```python
from build123d import *
from build123d.topology import SkipClean

# Parameters (mm, degrees)
SKETCH_1_R          = 1.525
SKETCH_1_R_2        = 1.025
SKETCH_1_R_3        = 2.5
EXTRUDE_1_DEPTH     = 2
CUT_EXTRUDE_START   = -10
CUT_EXTRUDE_1_DEPTH = 10
EXTRUDE_START       = -2
EXTRUDE_2_DEPTH     = 2
FILLET_1_R          = 10


with BuildPart() as part:
    # 草图1 → 凸台-拉伸1 (new body)
    with BuildSketch(Plane.XY):
        with BuildLine():
            Line((-2.51867373, 21.028627098), (-3.989978187, 0.282973621))
            ThreePointArc((-3.989978187, 0.282973621), (-3.84073462, -1.117478224), (-3.215350618, -2.379394965))
            Line((-3.215350618, -2.379394965), (6.832036867, -15.956743003))
            ThreePointArc((6.832036867, -15.956743003), (9.5375, -16.519434577), (10.402926369, -13.895088987))
            Line((10.402926369, -13.895088987), (3.941503233, 0.966479061))
            Line((3.941503233, 0.966479061), (2.51867373, 21.028627098))
            ThreePointArc((2.51867373, 21.028627098), (0, 23.375), (-2.51867373, 21.028627098))
        make_face()
        with Locations((0, 20.85)):
            Circle(SKETCH_1_R, mode=Mode.SUBTRACT)
        with Locations((8.5, -14.722431864)):
            Circle(SKETCH_1_R_2, mode=Mode.SUBTRACT)
        Circle(SKETCH_1_R_3, mode=Mode.SUBTRACT)
    extrude(amount=EXTRUDE_1_DEPTH)

    # 草图2 → 切除-拉伸1 (cut)
    with SkipClean():  # the faces are left unmerged after this step: merging them gives an invalid solid
        with BuildSketch(Plane.XY.offset(2).offset(CUT_EXTRUDE_START)):
            with BuildLine():
                Line((-2.51867373, 21.028627098), (-3.989978187, 0.282973621))
                ThreePointArc((-3.989978187, 0.282973621), (-3.896440427, 0.904296412), (-3.706760113, 1.503306179))
                ThreePointArc((-3.706760113, 1.503306179), (-1.57526628, 10.762235027), (-2.446005808, 20.22335769))
                ThreePointArc((-2.446005808, 20.22335769), (-2.514781389, 20.623064846), (-2.51867373, 21.028627098))
            make_face()
        extrude(amount=CUT_EXTRUDE_1_DEPTH, mode=Mode.SUBTRACT)

    # 草图3 → 凸台-拉伸2 (add)
    with SkipClean():  # the faces are left unmerged after this step: merging them gives an invalid solid
        with BuildSketch(Plane.XY.offset(2).offset(EXTRUDE_START)):
            with BuildLine():
                Line((0, 4), (0, 18.325))
                ThreePointArc((0, 18.325), (2.105124017, 19.455698069), (2.324893847, 21.835136337))
                ThreePointArc((2.324893847, 21.835136337), (5.020381454, 10.519043648), (3.858239677, -1.055455635))
                ThreePointArc((3.858239677, -1.055455635), (3.179765914, 2.426744471), (0, 4))
            make_face()
        extrude(amount=EXTRUDE_2_DEPTH)

    # 圆角1
    fillet_1_edges = [part.edges().sort_by_distance(p)[0] for p in [
        (4.210891787, 0.346873093, 1),
    ]]
    fillet(fillet_1_edges, radius=FILLET_1_R)


solid = part.part
```
Verification items for the finished model (mm, model axes). Coordinates: 2 decimals unless noted, no trailing zeros. Write each loop counter-clockwise with the first axis right and the second up, starting at its lowest first coordinate (ties: lowest second). Pieces come first, ordered by that corner, then holes. Notation, with made-up numbers: M -12.75,-15 L 8.25,-15 A25 ccw 8.25,-1 Z; hole C 46,77 d3. An arc over 180 degrees is marked long. One line per item, written item: value.
Item 1: Section check D-D, the plane y = 7.5. Record the boundary of the cut face in (x, z).
Check sheet entries:
outline: M -1.98,0 L 5.09,0 L 5.09,2 L -1.98,2 Z
Item 2: Section check A-A, the plane x = 8. Record the boundary of the cut face in (y, z).
Check sheet entries:
outline: M -16.74,0 L -15.62,0 L -15.62,2 L -16.74,2 Z; M -13.83,0 L -8.37,0 L -8.37,2 L -13.83,2 Z
Item 3: Section check B-B, the plane x = 0. Record the boundary of the cut face in (y, z) (3 decimals), plus the area to 3 significant figures.
Check sheet entries:
outline: M -6.724,0 L -2.5,0 L -2.5,2 L -6.724,2 Z; M 2.5,0 L 19.325,0 L 19.325,2 L 2.5,2 Z; M 22.375,0 L 23.375,0 L 23.375,2 L 22.375,2 Z
area: 44.1 mm^2
Item 4: Scan lines: line 1 along Y through (x, z) = (-1, 0.45); line 2 along Y through (x, z) = (0, 0.65) (3 decimals); line 3 along X through (y, z) = (-1.5, 0.85). Record each from-to range of solid material in increasing order.
Check sheet entries:
line 1: y = -5.37 to -2.29, 2.29 to 19.7, 22 to 23.17
line 2: y = -6.724 to -2.5, 2.5 to 19.325, 22.375 to 23.375
line 3: x = -3.71 to -2, 2 to 5.07
Item 5: Mould release check, pull along Y, two halves, no side actions. Record for faces 1 (the flat face through (2, 4, 0)), 2 (the cylindrical face through (9.5, -16.54, 0.99)), 3 (the cylindrical face through (4.803, 12.717, 0.986)): pulls with the +Y half, pulls with the -Y half, needs draft (parallel to the pull), parting line crosses it, or undercut.
Check sheet entries:
face 1: needs draft
face 2: parting line crosses it
face 3: undercut
Item 6: Section check C-C, the plane z = 0.55. Record the boundary of the cut face in (x, y) (3 decimals), plus the area to 3 significant figures.
Check sheet entries:
outline: M -3.707,1.503 A4 ccw -3.215,-2.379 L 6.832,-15.957 A2.075 ccw 10.403,-13.895 L 5.433,-2.464 A10 cw 4.714,3.003 A35 ccw 2.325,21.835 A2.525 ccw -2.446,20.223 A30 cw Z; hole C 0,0 d5; hole C 0,20.85 d3.05; hole C 8.5,-14.722 d2.05
area: 231 mm^2
